Can you work these out from the drawing? Everything is in mm from the part's minimum corner. A direction names the side the tool comes from. Round coordinates to 2 decimals unless told otherwise and drop trailing zeros. Loops run counter-clockwise (first coordinate to the right, second up) from the corner with the lowest first, then second, coordinate; pieces in that order, holes last. Notation, with made-up numbers: (68.5, 36) - (110.5, 36) arc R8 ccw to (110.5, 44) - close; hole circle Ø2 at (20, 32.25). An arc over 180 degrees is marked (long way). Answer as CSV lines item,"result". Start each with the question number.
1) We'd pull the mould along Z, two halves only. Please class the marked faces 1, 2 and 3: pulls with the +Z half, pulls with the -Z half, needs draft (parallel to the pull), parting line crosses it, or undercut.
2) Which directions (+Z, -Z, +X, -X, +Y, -Y) give clear straight access to the entire face, cutting with the end or side of a thin tool? Please do the marked faces 4 and 5.
3) Suppose I cut it at A-A, the plane x = 12.7. Write out the boundary of the cut face in (y, z), then the cut area to 3 significant figures.
4) Suppose I cut it at D-D, the plane z = 12.7. Write out the boundary of the cut face in (x, y).
5) I'm going to push flat-ended pins straight in: pin 1 Ø1 at (x, y) = (46.5, 5) entering from +Z; pin 2 Ø10.5 at (x, z) = (31.75, 50.8) entering from +Y; pin 3 Ø3 at (x, y) = (41, 2) entering from -Z. Where does each tip first touch, or does it pass through?
6) Please list where these lines run through material, in increasing order: line 1 along X through (y, z) = (4.5, 31.75) (1 decimal); line 2 along Y through (x, z) = (32, 40); line 3 along Z through (x, y) = (15, 4.5) (1 decimal).
7) Suppose I cut it at B-B, the plane z = 31.75. Count the separate pieces of the cut face and the enclosed holes in it, then the cut area to 3 significant figures.
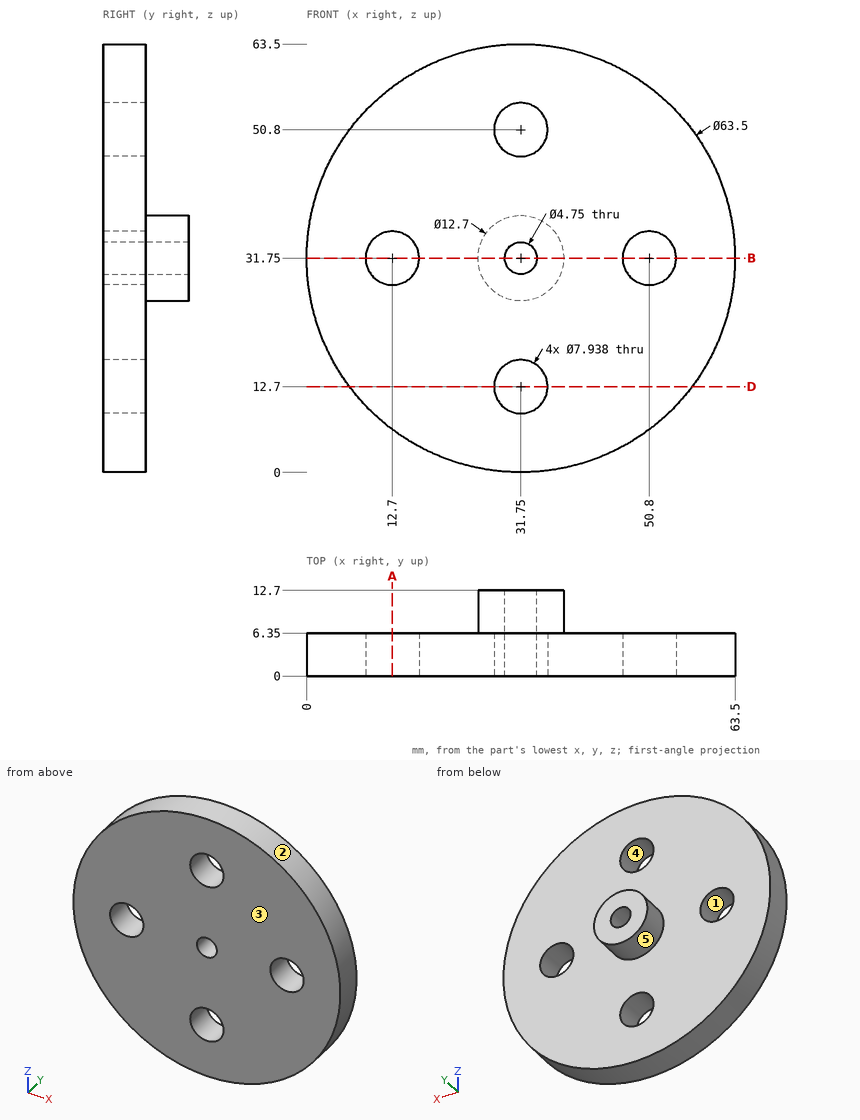
Filled sheet:
1,face 1,"undercut"
1,face 2,"parting line crosses it"
1,face 3,"needs draft"
2,face 4,"+Y, -Y"
2,face 5,"+Y"
3,outline,"(0, 6.35) - (6.35, 6.35) - (6.35, 27.78) - (0, 27.78) - close; (0, 35.72) - (6.35, 35.72) - (6.35, 57.15) - (0, 57.15) - close"
3,area,"272 mm²"
4,outline,"(6.35, 0) - (27.78, 0) - (27.78, 6.35) - (6.35, 6.35) - close; (35.72, 0) - (57.15, 0) - (57.15, 6.35) - (35.72, 6.35) - close"
5,pin 1,"z = 60.12"
5,pin 2,"y = 6.35"
5,pin 3,"z = 0.96"
6,line 1,"0 to 8.7, 16.7 to 29.4, 34.1 to 46.8, 54.8 to 63.5"
6,line 2,"0 to 6.35"
6,line 3,"4.8 to 28.5, 35 to 58.7"
7,separate pieces,"4"
7,enclosed holes,"0"
7,area,"323 mm²"
